Autodesk Inventor part; units mm, degrees
ref_plane "YZ Plane" through (0, 0, 0) normal (1, 0, 0) x (0, 1, 0)
ref_plane "XZ Plane" through (0, 0, 0) normal (0, 1, 0) x (-1, 0, 0)
ref_plane "XY Plane" through (0, 0, 0) normal (0, 0, 1) x (1, 0, 0)
sketch "Sketch1" plane through (0, 0, 0) normal (0, 1, 0) x (-1, 0, 0)
  line L0 (3, 0) -> (53, 0)
  line L1 (56, -3) -> (56, -82)
  line L2 (53, -85) -> (3, -85)
  line L3 (0, -82) -> (0, -3)
  arc A0 (56, -3) -> (53, 0) centre (53, -3) ccw
  arc A1 (53, -85) -> (56, -82) centre (53, -82) ccw
  arc A2 (0, -82) -> (3, -85) centre (3, -82) ccw
  arc A3 (3, 0) -> (0, -3) centre (3, -3) ccw
  point P0 (0, 0)
  point P1 (56, 0)
  point P2 (0, -85)
  dimension "d0" = 56
  dimension "d1" = 85
  dimension "d2" = 3
extrude "Extrusion1" add sketch "Sketch1" along normal blind 4
chamfer "Chamfer1" distance 2 angle 45 8 edges at (0, 4, -42.5) (-0.8787, 4, -84.1213) (-28, 4, -85) (-55.1213, 4, -84.1213) (-56, 4, -42.5) (-55.1213, 4, -0.8787) (-28, 4, 0) (-0.8787, 4, -0.8787)
sketch "Sketch2" plane through (0, 0, 0) normal (0, 1, 0) x (-1, 0, 0)
  line L0 (53, 0) -> (3, 0)
  line L1 (3, -85) -> (53, -85)
  line L2 (44.8, 0) -> (48.5333, 0)
  line L3 (48.5333, 0) -> (48.5333, -85)
  line L4 (48.5333, -85) -> (44.8, -85)
  line L5 (44.8, -85) -> (44.8, 0)
  line L6 (56, -82) -> (56, -3)
  line L7 (41.0667, 0) -> (44.8, 0)
  line L8 (44.8, 0) -> (44.8, -85)
  line L9 (44.8, -85) -> (41.0667, -85)
  line L10 (41.0667, -85) -> (41.0667, 0)
  line L11 (37.3334, 0) -> (41.0667, 0)
  line L12 (41.0667, 0) -> (41.0667, -85)
  line L13 (41.0667, -85) -> (37.3334, -85)
  line L14 (37.3334, -85) -> (37.3334, 0)
  line L15 (33.6001, 0) -> (37.3334, 0)
  line L16 (37.3334, 0) -> (37.3334, -85)
  line L17 (37.3334, -85) -> (33.6001, -85)
  line L18 (33.6001, -85) -> (33.6001, 0)
  line L19 (29.8668, 0) -> (33.6001, 0)
  line L20 (33.6001, 0) -> (33.6001, -85)
  line L21 (33.6001, -85) -> (29.8668, -85)
  line L22 (29.8668, -85) -> (29.8668, 0)
  line L23 (26.1335, 0) -> (29.8668, 0)
  line L24 (29.8668, 0) -> (29.8668, -85)
  line L25 (29.8668, -85) -> (26.1335, -85)
  line L26 (26.1335, -85) -> (26.1335, 0)
  line L27 (22.4002, 0) -> (26.1335, 0)
  line L28 (26.1335, 0) -> (26.1335, -85)
  line L29 (26.1335, -85) -> (22.4002, -85)
  line L30 (22.4002, -85) -> (22.4002, 0)
  line L31 (18.6669, 0) -> (22.4002, 0)
  line L32 (22.4002, 0) -> (22.4002, -85)
  line L33 (22.4002, -85) -> (18.6669, -85)
  line L34 (18.6669, -85) -> (18.6669, 0)
  line L35 (14.9336, 0) -> (18.6669, 0)
  line L36 (18.6669, 0) -> (18.6669, -85)
  line L37 (18.6669, -85) -> (14.9336, -85)
  line L38 (14.9336, -85) -> (14.9336, 0)
  line L39 (11.2003, 0) -> (14.9336, 0)
  line L40 (14.9336, 0) -> (14.9336, -85)
  line L41 (14.9336, -85) -> (11.2003, -85)
  line L42 (11.2003, -85) -> (11.2003, 0)
  line L43 (7.467, 0) -> (11.2003, 0)
  line L44 (11.2003, 0) -> (11.2003, -85)
  line L45 (11.2003, -85) -> (7.467, -85)
  line L46 (7.467, -85) -> (7.467, 0)
  point P0 (0, 0)
  dimension "d8" = 7.4667
  dimension "d9" = 3.7333
  dimension "d12" = 3.7333
extrude "Extrusion2" cut sketch "Sketch2" against normal blind 2 from surface at 4 contours L3 L1 L5 L0 | L10 L1 L14 L0 | L18 L1 L22 L0 | L26 L1 L30 L0 | L34 L1 L38 L0 | L42 L1 L46 L0
sketch "Sketch3" plane through (0, 0, 0) normal (0, -1, 0) x (1, 0, 0)
  line L0 (-3, 0) -> (-5.85, 0)
  line L1 (-5.85, 0) -> (-5.85, -3)
  line L2 (-2.85, -6) -> (0, -6)
  line L3 (0, -6) -> (0, -3)
  line L4 (0, -3) -> (0, -82)
  line L5 (0, -58.5) -> (-4.467, -58.5)
  line L6 (-5.85, -64.5) -> (-5.85, -64.5)
  line L7 (-4.467, -64.5) -> (0, -64.5)
  line L8 (0, -64.5) -> (0, -58.5)
  line L9 (-28, 0) -> (-28, -85) construction
  line L10 (-53, 0) -> (-3, 0)
  line L11 (-3, -85) -> (-53, -85)
  arc A0 (0, -3) -> (-3, 0) centre (-3, -3) ccw
  arc A1 (-5.85, -3) -> (-2.85, -6) centre (-2.85, -3) ccw
  line L12 (0, -6) -> (-5.85, -6)
  line L13 (0, -58.5) -> (-2.85, -58.5)
  line L14 (-2.85, -64.5) -> (0, -64.5)
  line L15 (-5.85, -61.5) -> (-5.85, -61.5)
  arc A2 (-2.85, -58.5) -> (-5.85, -61.5) centre (-2.85, -61.5) ccw
  arc A3 (-5.85, -61.5) -> (-2.85, -64.5) centre (-2.85, -61.5) ccw
  line L16 (0, -58.5) -> (-5.85, -58.5)
  line L17 (-5.85, -58.5) -> (-5.85, -64.5)
  line L18 (-5.85, -64.5) -> (0, -64.5)
  line L19 (0, -3) -> (0, -82)
  line L20 (-5.85, -6) -> (-5.85, 0)
  line L21 (-53, 0) -> (-50.15, 0)
  line L22 (-50.15, 0) -> (-50.15, -3)
  line L23 (-53.15, -6) -> (-56, -6)
  line L24 (-56, -6) -> (-56, -3)
  line L25 (-56, -58.5) -> (-51.533, -58.5)
  line L26 (-50.15, -64.5) -> (-50.15, -64.5)
  line L27 (-51.533, -64.5) -> (-56, -64.5)
  line L28 (-56, -64.5) -> (-56, -58.5)
  arc A4 (-53, 0) -> (-56, -3) centre (-53, -3) ccw
  arc A5 (-53.15, -6) -> (-50.15, -3) centre (-53.15, -3) ccw
  line L29 (-56, -6) -> (-50.15, -6)
  line L30 (-56, -58.5) -> (-53.15, -58.5)
  line L31 (-53.15, -64.5) -> (-56, -64.5)
  line L32 (-50.15, -61.5) -> (-50.15, -61.5)
  arc A6 (-50.15, -61.5) -> (-53.15, -58.5) centre (-53.15, -61.5) ccw
  arc A7 (-53.15, -64.5) -> (-50.15, -61.5) centre (-53.15, -61.5) ccw
  line L33 (-56, -58.5) -> (-50.15, -58.5)
  line L34 (-50.15, -58.5) -> (-50.15, -64.5)
  line L35 (-50.15, -64.5) -> (-56, -64.5)
  line L36 (-50.15, -6) -> (-50.15, 0)
  point P0 (0, 0)
  point P1 (-7.467, 0)
  point P2 (-2.2335, -58.5)
  point P3 (0, -64.5)
  point P4 (-7.467, -2)
  point P5 (-56, 0)
  point P6 (-48.533, 0)
  point P7 (-56, -3)
  point P8 (-53.7665, -58.5)
  point P9 (-53, 0)
  point P10 (-48.533, -2)
  point P11 (-53.15, -58.5)
  point P12 (-5.85, -61.5)
  point P13 (-2.85, -64.5)
  point P14 (-2.85, -58.5)
  point P15 (-50.15, 0)
  point P16 (-2.85, -6)
  dimension "d19" = 6
  dimension "d21" = 58.5
  dimension "d22" = 6
  dimension "d25" = 28
  dimension "d26" = 3
  dimension "d29" = 3
  dimension "d30" = 3
  dimension "d48" = 5.85
extrude "Extrusion3" add sketch "Sketch3" along normal blind 3 contours A0 L3 L2 A1 L1 L0 | L4 L7 A3 A2 L5 | L22 A5 L23 L24 A4 L10 | L25 A6 A7 L27 L28
extrude "Extrusion4" cut sketch "Sketch3" along normal blind 2 from surface at -4 contours A0 L3 L2 A1 L1 L0 | L4 L7 A3 A2 L5 | L22 A5 L23 L24 A4 L10 | L36 L29 A5 | A2 L17 L16 L5 | L7 L18 L17 A3 | L25 A6 A7 L27 L28 | L25 L33 L34 A6 | L34 L35 L27 A7
sketch "Sketch4" plane through (-53, 2, 0) normal (0, 1, 0) x (1, 0, 0)
  line L0 (-0.15, 58.5) -> (-3, 58.5)
  line L1 (-3, 64.5) -> (-3, 58.5)
  line L2 (-3, 6) -> (-3, 3)
  line L3 (0, 0) -> (2.85, 0)
  line L4 (47.15, 0) -> (50, 0)
  line L5 (53, 3) -> (53, 6)
  line L6 (53, 58.5) -> (53, 64.5)
  line L7 (50.15, 64.5) -> (53, 64.5)
  point P0 (0.5, 3.5)
  point P1 (0.5, 61.5)
  point P2 (49.5, 61.5)
  point P3 (49.5, 3.5)
  dimension "d49" = 3
  dimension "d50" = 3.5
  dimension "d51" = 3.5
  dimension "d52" = 3.5
  dimension "d53" = 3.5
  dimension "d54" = 3.5
  dimension "d55" = 3.5
  dimension "d56" = 3
hole "Hole1" at (-52.5, 2, -3.5) at (-52.5, 2, -61.5) at (-3.5, 2, -61.5) at (-3.5, 2, -3.5) direction (0, -1, 0) diameter 2.7 end through all
properties part number "Raspberry-Pi-4B heatsink1" material "Aluminum 6061"
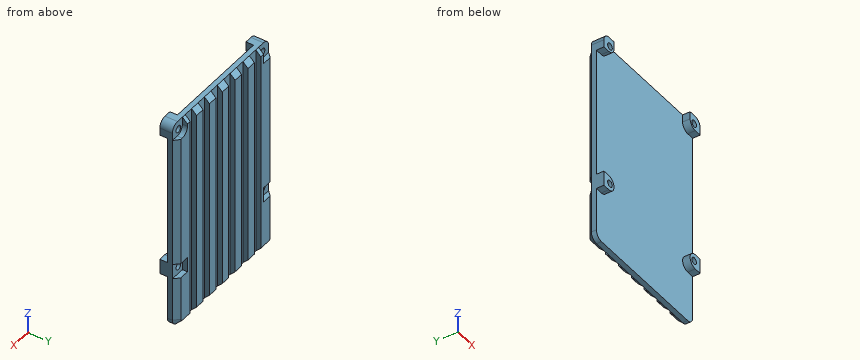
Could you check a few things on this model? Use its own coordinates, in mm. Coordinates: 2 decimals unless noted, no trailing zeros. Loops run counter-clockwise (first coordinate to the right, second up) from the corner with the lowest first, then second, coordinate; pieces in that order, holes last. Notation, with made-up numbers: (62, 2) -> (87, 2) arc R20 cw to (87, 27) -> close; hole circle Ø3 at (-16.5, -29.75). An arc over 180 degrees is marked (long way). Answer in a Markdown table with one row per item.
(1) Will these pins go through, and if not, where does the flat tip stop? pin 1 Ø3 at (y, z) = (-2, -50.5) entering from -X; pin 2 Ø2 at (x, y) = (-54.5, 3) entering from -Z; pin 3 Ø2 at (x, z) = (-10.5, -29) entering from -Y; pin 4 Ø1 at (x, y) = (-1, 3.5) entering from +Z.
Results found:
| item | result |
|---|---|
| pin 1 | passes through |
| pin 2 | stops at z = -84.7 |
| pin 3 | stops at y = 0 |
| pin 4 | stops at z = -6 |
(2) Imagine slicing it at C-C (x = -32.5). List the corners of the cut face in (y, z) for me.
Results found:
| item | result |
|---|---|
| outline | (0, -85) -> (2, -85) -> (2, 0) -> (0, 0) -> close |
(3) If I drill on probe 1 along X at (y, z) = (-0.35, -61.5); probe 2 along Z at (x, y) = (-52.5, 0.2); probe 3 along Z at (x, y) = (-3.5, -1.7), over which ranges is the centre line in solid material (lowest first)?
Results found:
| item | result |
|---|---|
| probe 1 | x = -56 to -53.85, -51.15 to -50.15, -5.85 to -4.85, -2.15 to 0 |
| probe 2 | z = -85 to -62.85, -60.15 to -4.85, -2.15 to 0 |
| probe 3 | z = -64.43 to -62.85, -60.15 to -58.57, -5.93 to -4.85, -2.15 to 0 |
(4) Imagine slicing it at A-A (y = -1.5). List the corners of the cut face in (x, z) for me, plus the area to 3 significant figures.
Results found:
| item | result |
|---|---|
| outline | (-56, -64.5) -> (-53.15, -64.5) arc R3 ccw to (-53.15, -58.5) -> (-56, -58.5) -> close; (-56, -6) -> (-53.15, -6) arc R3 ccw to (-50.15, -3) -> (-50.15, 0) -> (-53, 0) arc R3 ccw to (-56, -3) -> close; (-5.85, -3) arc R3 ccw to (-2.85, -6) -> (0, -6) -> (0, -3) arc R3 ccw to (-3, 0) -> (-5.85, 0) -> close; (-2.85, -64.5) -> (0, -64.5) -> (0, -58.5) -> (-2.85, -58.5) arc R3 ccw to start; hole circle Ø2.7 at (-52.5, -61.5); hole circle Ø2.7 at (-52.5, -3.5); hole circle Ø2.7 at (-3.5, -61.5); hole circle Ø2.7 at (-3.5, -3.5) |
| area | 102 mm^2 |
